Autodesk Inventor part; units mm, degrees
ref_plane "YZ Plane" through (0, 0, 0) normal (1, 0, 0) x (0, 1, 0)
ref_plane "XZ Plane" through (0, 0, 0) normal (0, 1, 0) x (-1, 0, 0)
ref_plane "XY Plane" through (0, 0, 0) normal (0, 0, 1) x (1, 0, 0)
sketch "Skizze1" plane through (0, 0, 0) normal (0, 1, 0) x (-1, 0, 0)
  line L0 (25.085, 0) -> (-63.4246, 0)
  line L1 (0, 50.1146) -> (0, -66.9502)
  line L2 (15, 15) -> (-15, 15)
  line L3 (-15, 15) -> (-15, -15)
  line L4 (-15, -15) -> (15, -15)
  line L5 (15, -15) -> (15, 15)
  line L6 (15, 15) -> (-15, -15) construction
  line L7 (-15, 15) -> (15, -15) construction
  circle A0 centre (0, 0) radius 2
  dimension "d0" = 30
  dimension "d1" = 30
  dimension "d24" = 4
extrude "Extrusion1" add sketch "Skizze1" along normal blind 130
sketch "Skizze3" plane through (0, 130, 0) normal (0, 1, 0) x (1, 0, 0)
  line L0 (18.5438, 0) -> (-21.4353, 0) construction
  line L1 (-11, 7.5) -> (-11, -7.5)
  line L2 (-15, 15) -> (-15, -15)
  line L3 (15, 15) -> (-15, 15)
  line L4 (-11, 7.5) -> (-15, 3.5)
  line L5 (-11, -7.5) -> (-15, -3.5)
  line L6 (-15.2121, -3.7121) -> (-10.7, -8.2243)
  line L7 (-10.7, -8.2243) -> (-10.7, 8.2243)
  line L8 (-10.7, 8.2243) -> (-15.2121, 3.7121)
  line L9 (-15, -3.9243) -> (-15, 3.9243)
  line L10 (3.7121, -15.2121) -> (8.2243, -10.7)
  line L11 (8.2243, -10.7) -> (-8.2243, -10.7)
  line L12 (-8.2243, -10.7) -> (-3.7121, -15.2121)
  line L13 (3.9243, -15) -> (-3.9243, -15)
  line L14 (15.2121, 3.7121) -> (10.7, 8.2243)
  line L15 (10.7, 8.2243) -> (10.7, -8.2243)
  line L16 (10.7, -8.2243) -> (15.2121, -3.7121)
  line L17 (15, 3.9243) -> (15, -3.9243)
  line L18 (-3.7121, 15.2121) -> (-8.2243, 10.7)
  line L19 (-8.2243, 10.7) -> (8.2243, 10.7)
  line L20 (8.2243, 10.7) -> (3.7121, 15.2121)
  line L21 (-3.9243, 15) -> (3.9243, 15)
  point P0 (0, 0)
  point P1 (3.9243, 15)
  point P2 (-3.9243, 15)
  dimension "d11" = 4
  dimension "d12" = 15
  dimension "d13" = 7.5
  dimension "d14" = 45
  dimension "d15" = 45
  dimension "d18" = 0.3
  dimension "d22" = 360
extrude "Extrusion3" cut sketch "Skizze3" against normal blind 30
fillet "Rundung1" radius 0.2 2 edges at (-15, 115, 3.9243) (-15, 115, -3.9243)
extrude "Extrusion4" cut sketch "Skizze1" along normal blind 6.7 contours A0 L1 L0 | L0 L1 A0 | L1 A0 L0 | L0 A0 L1
properties part number "CarlaRescueRampeTeil1"
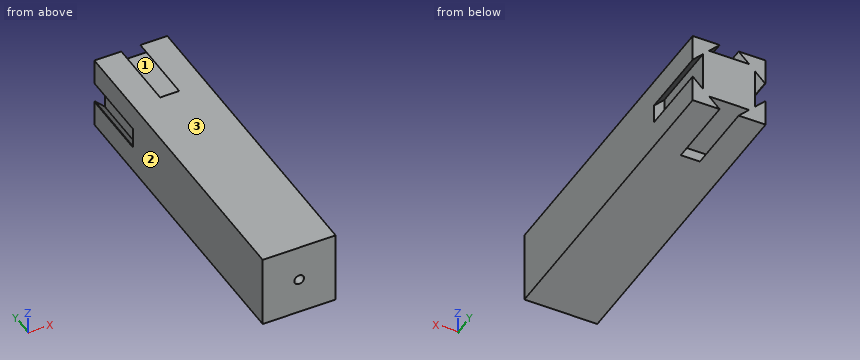
Geometry check sheet. Reference: the model listing, model coordinates, mm. Face numbers are marked on the shaded views. Round coordinates to 2 decimals unless told otherwise and drop trailing zeros. Write each loop counter-clockwise with the first axis right and the second up, starting at its lowest first coordinate (ties: lowest second). Pieces come first, ordered by that corner, then holes. Notation, with made-up numbers: (31.25, 86) -> (43.25, 86) arc R27 cw to (43.25, 123) -> close; hole circle Ø9 at (-36.75, 72.5). An arc over 180 degrees is marked (long way). One line per item, written item: value. Start each with the question number.
(1) Cross-section at C-C, the plane y = 111. Record the cut outline in (x, z), and give its area (3 significant figures).
(2) Scan lines: line 1 (X direction, y = 2.5, z = 0); line 2 (X direction, y = 124.5, z = -8). Record each from-to range of solid material in increasing order. Write a range as [from, to].
(3) Draft check along Z on the marked faces 1, 2 and 3. Enter one of: +Z half, -Z half, draft (parallel to the pull), parting line (faces both ways), or undercut.
(4) Cross-section at B-B, the plane x = 0. Record the cut outline in (y, z), and give its area (3 significant figures).
(5) Cross-section at A-A, the plane z = 0. Record the cut outline in (x, y).
(6) Go/stop test with a flat-tipped pin: pin 1 Ø1.3 at (x, z) = (3.5, 13) entering from +Y. Record where the tip stops, or that it passes through.
(7) Cross-section at D-D, the plane z = 12. Record the cut outline in (x, y), and give its area (3 significant figures).
Answer:
1. outline: (-15, -15) -> (-3.92, -15) -> (-8.22, -10.7) -> (8.22, -10.7) -> (3.92, -15) -> (15, -15) -> (15, -3.92) -> (10.7, -8.22) -> (10.7, 8.22) -> (15, 3.92) -> (15, 15) -> (3.92, 15) -> (8.22, 10.7) -> (-8.22, 10.7) -> (-3.92, 15) -> (-15, 15) -> (-15, 4.41) arc R0.2 ccw to (-14.66, 4.27) -> (-10.7, 8.22) -> (-10.7, -8.22) -> (-14.66, -4.27) arc R0.2 ccw to (-15, -4.41) -> close
1. area: 691 mm²
2. line 1: [-15, -2], [2, 15]
2. line 2: [-15, -10.92], [-10.7, 10.7], [10.92, 15]
3. face 1: undercut
3. face 2: draft
3. face 3: +Z half
4. outline: (0, -15) -> (100, -15) -> (100, -10.7) -> (130, -10.7) -> (130, 10.7) -> (100, 10.7) -> (100, 15) -> (0, 15) -> (0, 2) -> (6.7, 2) -> (6.7, -2) -> (0, -2) -> close
4. area: 3,620 mm²
5. outline: (-15, 0) -> (-2, 0) -> (-2, 6.7) -> (2, 6.7) -> (2, 0) -> (15, 0) -> (15, 100) -> (10.7, 100) -> (10.7, 130) -> (-10.7, 130) -> (-10.7, 100) -> (-15, 100) -> close
6. pin 1: y = 100
7. outline: (-15, 0) -> (15, 0) -> (15, 130) -> (6.92, 130) -> (6.92, 100) -> (-6.92, 100) -> (-6.92, 130) -> (-15, 130) -> close
7. area: 3,480 mm²
